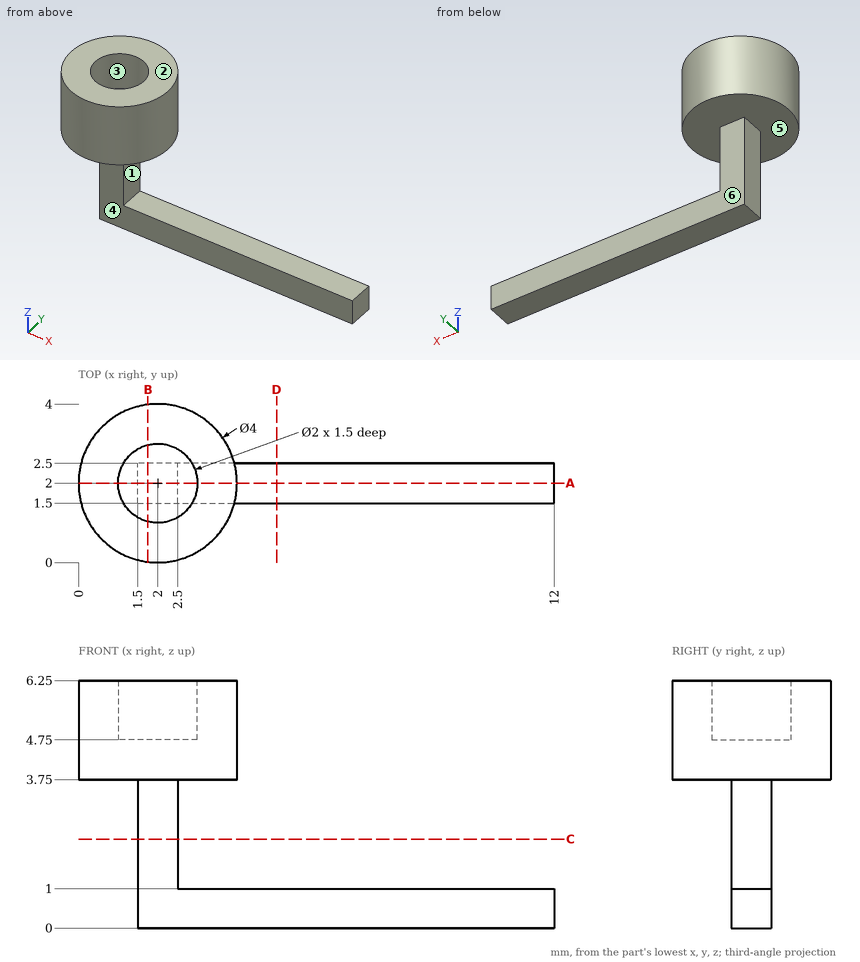
The drawing under review shows one solid part. Ordinate dimensions are in mm from its lowest x, y, z. A direction names the side the tool comes from. Give positions to 0.01 mm unless a question says otherwise; leave off trailing zeros. Order: outer loops, then holes, each group sorted by start corner. A loop starts at its lowest first (then second) coordinate and runs counter-clockwise, first axis right, second up. Notation, with made-up numbers: (60, -21.75) - (87, -21.75) arc R30 cw to (87, 1.25) - close; hole circle Ø8 at (69, 55.5). An arc over 180 degrees is marked (long way). Answer as a JSON object with one key per item and string values. Group by question number.
Item 1: Take a section at C-C on z = 2.25. Give the boundary of the cut face in (x, y).
Item 2: Machinability: for the marked faces 4, 5 and 6, which of the approach directions +Z, -Z, +X, -X, +Y, -Y give a long, thin tool a straight path to every point of the face, cutting with its end or side? Answer none if there is none.
Item 3: Take a section at D-D on x = 5. Give the boundary of the cut face in (y, z), and give its area (3 significant figures).
Item 4: Clearance check with flat-ended pins moving along their axes: pin 1 Ø2 at (x, y) = (2, 1.5) entering from +Z; pin 2 Ø1.5 at (y, z) = (2, 2.5) entering from -X; pin 3 Ø1.9 at (x, z) = (7.5, 1.5) entering from +Y; pin 4 Ø2 at (y, z) = (2, 3.5) entering from +X. State where each tip first meets the part, or that it passes through.
Item 5: Wall thickness on line 1 along Z through (x, y) = (3, 2.45); line 2 along Y through (x, z) = (2, 5.25); line 3 along Z through (x, y) = (5.25, 1.7): over which ranges is each line inside the solid? List them lowest first.
Item 6: Draft analysis for pull direction Z (two halves, no side actions). For the marked faces 1, 2 and 3, state which applies: pulls with the +Z half, pulls with the -Z half, needs draft (parallel to the pull), parting line crosses it, or undercut.
Item 7: Take a section at B-B on x = 1.75. Give the boundary of the cut face in (y, z).
Item 8: Take a section at A-A on y = 2. Give the boundary of the cut face in (x, z).
Reported:
{
 "1": {"outline": "(1.5, 1.5) - (2.5, 1.5) - (2.5, 2.5) - (1.5, 2.5) - close"},
 "2": {"face 4": "-Z, +X, -X, -Y", "face 5": "none", "face 6": "-Z, +X, -X, +Y"},
 "3": {"outline": "(1.5, 0) - (2.5, 0) - (2.5, 1) - (1.5, 1) - close", "area": "1.00 mm^2"},
 "4": {"pin 1": "z = 6.25", "pin 2": "x = 1.5", "pin 3": "y = 2.5", "pin 4": "x = 4"},
 "5": {"line 1": "0 to 1, 3.75 to 6.25", "line 2": "0 to 1, 3 to 4", "line 3": "0 to 1"},
 "6": {"face 1": "undercut", "face 2": "pulls with the +Z half", "face 3": "needs draft"},
 "7": {"outline": "(0.02, 3.75) - (1.5, 3.75) - (1.5, 0) - (2.5, 0) - (2.5, 3.75) - (3.98, 3.75) - (3.98, 6.25) - (2.97, 6.25) - (2.97, 4.75) - (1.03, 4.75) - (1.03, 6.25) - (0.02, 6.25) - close"},
 "8": {"outline": "(0, 3.75) - (1.5, 3.75) - (1.5, 0) - (12, 0) - (12, 1) - (2.5, 1) - (2.5, 3.75) - (4, 3.75) - (4, 6.25) - (3, 6.25) - (3, 4.75) - (1, 4.75) - (1, 6.25) - (0, 6.25) - close"}
}
